The model under review builds one solid part; all positions refer to its coordinate system, in mm. A direction names the side the tool comes from. Round coordinates to 2 decimals unless told otherwise and drop trailing zeros. Write each loop counter-clockwise with the first axis right and the second up, starting at its lowest first coordinate (ties: lowest second). Pieces come first, ordered by that corner, then holes. Notation, with made-up numbers: M 7.5,1 L 48.5,1 A23 ccw 48.5,17 Z; hole C 55,-15.5 d5. An arc over 180 degrees is marked long. One line per item, written item: value. Start each with the question number.
1) Tool access review of faces 4 (the face through (-2.2, 3.73, -1.48)), 5 (the face through (-0.867, 3.905, 3.451)): name each direction out of +Z, -Z, +X, -X, +Y, -Y from which nothing blocks a thin tool from reaching the whole face with its end or side.
2) For P1, Ø3, axis at x = -0.5, y = -4, coming from the +Z side, flat-tipped, find the tip position at first contact; note if it passes through.
3) Take a section at B-B, the plane y = 0. Write out the cut boundary in (x, z), and give its area (3 significant figures).
4) Take a section at A-A, the plane z = -1.25. Write out the cut boundary in (x, y).
5) Take a section at D-D, the plane y = -3.25. Write out the cut boundary in (x, z), and give its area (3 significant figures).
6) Mouldability with a two-part tool opening along X and no side actions: class faces 1 (the face through (2.44, 0.54, 1.93)), 2 (the face through (-2.13, -3.77, -1.48)), 3 (the face through (2, 2, 7)) as +X half, -X half, draft (parallel to the pull), parting line (faces both ways), or undercut.
7) Take a section at C-C, the plane x = -1. Write out the cut boundary in (y, z), and give its area (3 significant figures).
8) Wall thickness on probe 1 along Y at (x, z) = (0, 1.25); probe 2 along X at (y, z) = (0, -0.5); probe 3 along Z at (x, y) = (4, -1): over which ranges is each line inside the solid? List them lowest first.
Autodesk Inventor part; units mm, degrees
ref_plane "YZ Plane" through (0, 0, 0) normal (1, 0, 0) x (0, 1, 0)
ref_plane "XZ Plane" through (0, 0, 0) normal (0, 1, 0) x (-1, 0, 0)
ref_plane "XY Plane" through (0, 0, 0) normal (0, 0, 1) x (1, 0, 0)
sketch "Sketch1" plane through (0, 0, 0) normal (0, 0, 1) x (1, 0, 0)
  line L0 (0, 5) -> (4.3301, 2.5)
  line L1 (4.3301, 2.5) -> (4.3301, -2.5)
  line L2 (4.3301, -2.5) -> (0, -5)
  line L3 (0, -5) -> (-4.3301, -2.5)
  line L4 (-4.3301, -2.5) -> (-4.3301, 2.5)
  line L5 (-4.3301, 2.5) -> (0, 5)
  point P0 (0, 0)
  point P1 (0, 0)
  dimension "d0" = 10
extrude "Extrusion1" add sketch "Sketch1" against normal blind 3
sketch "Sketch2" plane through (0, 0, 0) normal (0, 0, 1) x (1, 0, 0)
  circle A0 centre (0, 0) radius 4
  dimension "d3" = 8
extrude "Extrusion2" add sketch "Sketch2" along normal blind 7
sketch "Sketch3" plane through (0, 0, 7) normal (0, 0, 1) x (1, 0, 0)
  circle A0 centre (0, 0) radius 4
hole "Hole1" at (0, 0, 7) direction (0, 0, -1) diameter 5 depth 10
thread "Thread1"
properties part number "156 part 2" material "Gold"
Checked values:
1. face 4: +Z, -Z, -X, +Y
1. face 5: +Z
2. P1: stops at z = 7
3. outline: M -4.33,-3 L -2.5,-3 L -2.5,7 L -4,7 L -4,0 L -4.33,0 Z; M 2.5,-3 L 4.33,-3 L 4.33,0 L 4,0 L 4,7 L 2.5,7 Z
3. area: 32.0 mm2
4. outline: M -4.33,-2.5 L 0,-5 L 4.33,-2.5 L 4.33,2.5 L 0,5 L -4.33,2.5 Z; hole C 0,0 d5
5. outline: M -3.03,-3 L 3.03,-3 L 3.03,0 L 2.33,0 L 2.33,7 L -2.33,7 L -2.33,0 L -3.03,0 Z
5. area: 50.8 mm2
6. face 1: undercut
6. face 2: -X half
6. face 3: draft
7. outline: M -4.42,-3 L -2.29,-3 L -2.29,7 L -3.87,7 L -3.87,0 L -4.42,0 Z; M 2.29,-3 L 4.42,-3 L 4.42,0 L 3.87,0 L 3.87,7 L 2.29,7 Z
7. area: 34.9 mm2
8. probe 1: y = -4 to -2.5, 2.5 to 4
8. probe 2: x = -4.33 to -2.5, 2.5 to 4.33
8. probe 3: z = -3 to 0
